Answer from the drawing. Dimensions are ordinates in mm from the lowest x, y and z of the part. A direction names the side the tool comes from. Coordinates: 2 decimals unless noted, no trailing zeros. Loops run counter-clockwise (first coordinate to the right, second up) from the corner with the lowest first, then second, coordinate; pieces in that order, holes last. Notation, with made-up numbers: (80, -37) - (111, -37) arc R29 cw to (111, -7) - close; hole circle Ø5 at (-18, -17.5). An arc over 180 degrees is marked (long way). One line per question, with ' | ' between items. Start each with the question number.
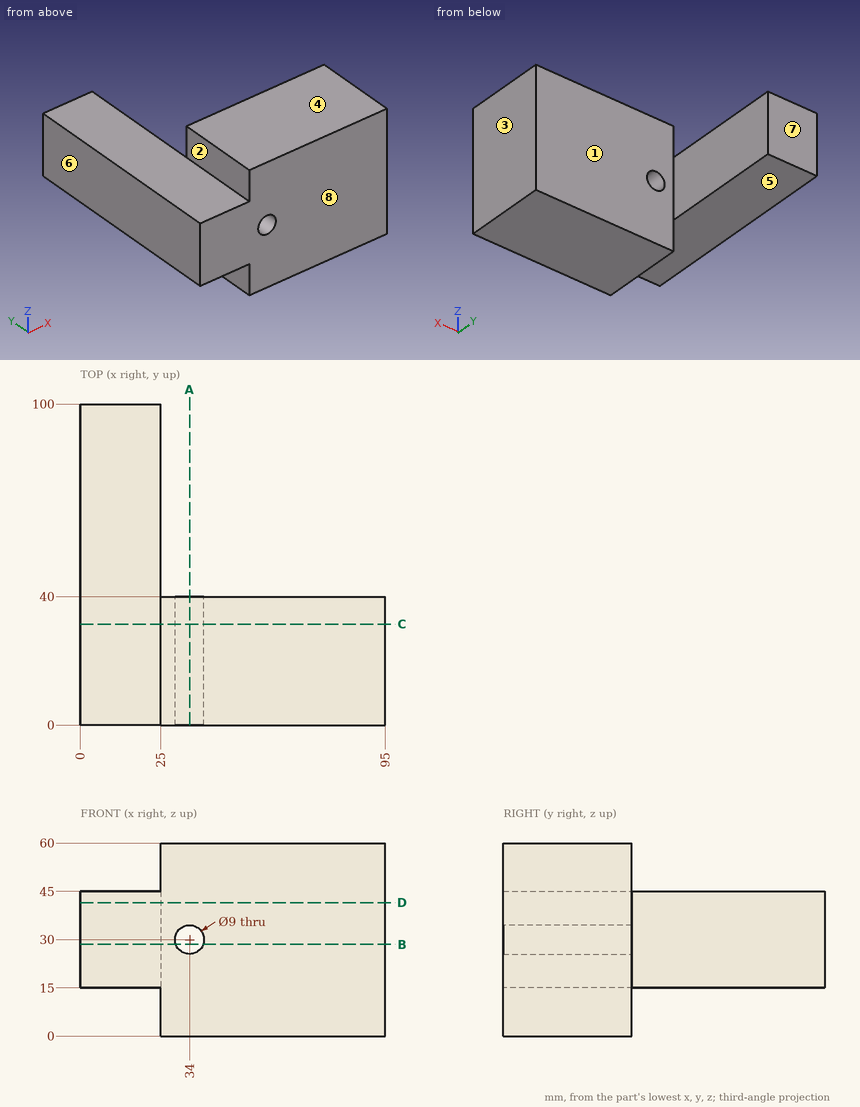
1) Given pin 1 Ø18 at (x, z) = (59, 29) entering from +Y; pin 2 Ø12.5 at (x, y) = (9, 33) entering from +Z; pin 3 Ø6 at (x, y) = (16.5, 39.5) entering from -Z, each flat-ended and moving along its own axis, determine where each tip first touches the part or whether it passes through.
2) The part is cut by section C-C on y = 31.5. Write down the section's boundary in (x, z), and give its area (3 significant figures).
3) Which of the six approach directions +Z, -Z, +X, -X, +Y, -Y give full straight-line access (tool end or side, diameter ignored) to the marked faces 1, 2, 3, 4 and 5?
4) The part is cut by section B-B on z = 28.5. Write down the section's boundary in (x, y), and give its area (3 significant figures).
5) The mould has two halves that part along Y. Classify the marked faces 6, 7 and 8: released by +Y, released by -Y, zero draft, split by the parting line, or undercut.
6) The part is cut by section D-D on z = 41.5. Write down the section's boundary in (x, y), and give its area (3 significant figures).
7) The part is cut by section A-A on x = 34. Write down the section's boundary in (y, z), and give its area (3 significant figures).
8) Find the intervals of material crossed by line 1 along X through (y, z) = (10, 30); line 2 along X through (y, z) = (24.5, 3.5); line 3 along Y through (x, z) = (62, 36.5), in increasing order. Write a range as from..to.
Answer below:
1) pin 1: y = 40 | pin 2: z = 45 | pin 3: z = 15
2) outline: (0, 15) - (25, 15) - (25, 0) - (95, 0) - (95, 60) - (25, 60) - (25, 45) - (0, 45) - close; hole circle Ø9 at (34, 30) | area: 4,890 mm2
3) face 1: +Z, -Z, +X, +Y | face 2: +Z, -X, +Y, -Y | face 3: +Z, -Z, +X, +Y, -Y | face 4: +Z, +X, -X, +Y, -Y | face 5: -Z, -X, +Y, -Y
4) outline: (0, 0) - (29.76, 0) - (29.76, 40) - (25, 40) - (25, 100) - (0, 100) - close; (38.24, 0) - (95, 0) - (95, 40) - (38.24, 40) - close | area: 4,960 mm2
5) face 6: zero draft | face 7: released by +Y | face 8: released by -Y
6) outline: (0, 0) - (95, 0) - (95, 40) - (25, 40) - (25, 100) - (0, 100) - close | area: 5,300 mm2
7) outline: (0, 0) - (40, 0) - (40, 25.5) - (0, 25.5) - close; (0, 34.5) - (40, 34.5) - (40, 60) - (0, 60) - close | area: 2,040 mm2
8) line 1: 0..29.5, 38.5..95 | line 2: 25..95 | line 3: 0..40
